For this review, use the dimensioned drawing (mm, ordinates from the lowest corner) and the shaded views. Round coordinates to 2 decimals unless told otherwise and drop trailing zeros. Order: outer loops, then holes, each group sorted by start corner. A loop starts at its lowest first (then second) coordinate and runs counter-clockwise, first axis right, second up. Notation, with made-up numbers: M 44.5,-4.75 L 78.5,-4.75 A24 ccw 78.5,18.25 Z; hole C 62,70.5 d10. An arc over 180 degrees is marked long. One line per item, written item: value. Start each with the question number.
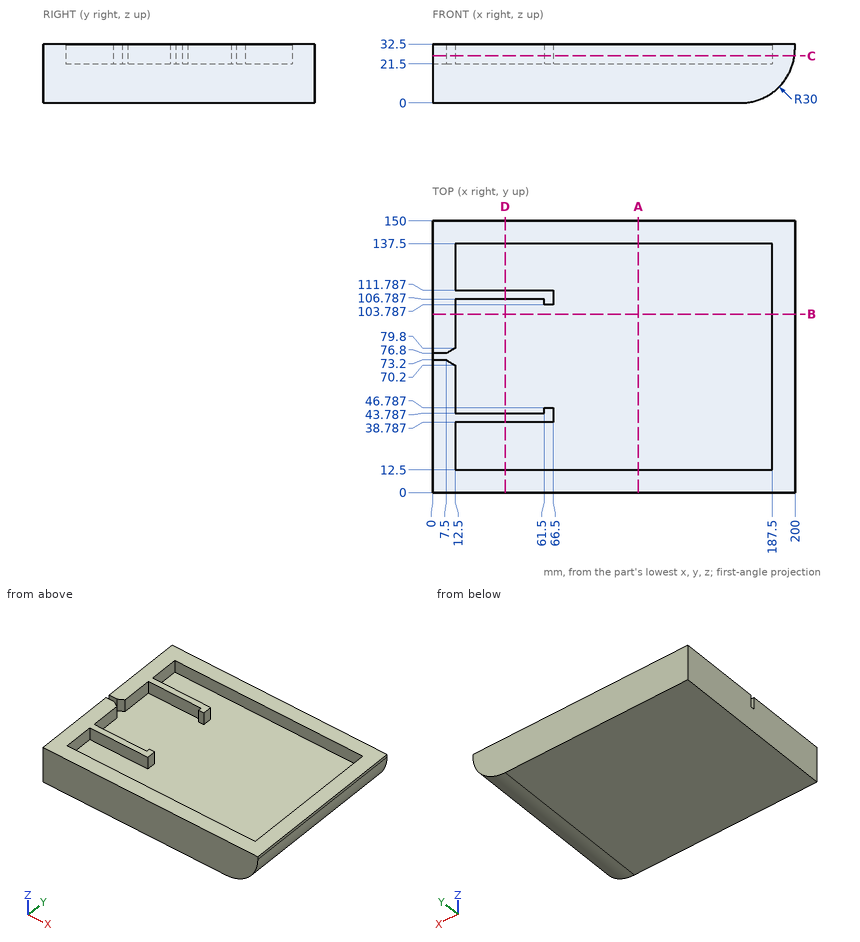
Item 1: Consider section D-D, the plane x = 40. Give the boundary of the cut face in (y, z), then the cut area to 3 significant figures.
Item 2: Clearance check with flat-ended pins moving along their axes: P1, Ø3.5, axis at y = 100, z = 24.5, coming from the +X side (1 decimal); P2, Ø3.5, axis at y = 55.5, z = 27.5, coming from the +X side; P3, Ø5.5, axis at y = 26, z = 25, coming from the +X side. State where each tip first meets the part, or that it passes through.
Item 3: Consider section A-A, the plane x = 113.5. Give the boundary of the cut face in (y, z).
Item 4: Consider section B-B, the plane y = 98.5. Give the boundary of the cut face in (x, z), then the cut area to 3 significant figures.
Item 5: Wall thickness on L1, parallel to Y at x = 50.5, z = 22.5; L2, parallel to Y at x = 64, z = 27.5; L3, parallel to X at y = 89, z = 29.5: over which ranges is each line inside the solid? List them lowest first.
Item 6: Consider section C-C, the plane z = 26. Give the boundary of the cut face in (x, y).
Computed:
1. outline: M 0,0 L 150,0 L 150,32.5 L 137.5,32.5 L 137.5,21.5 L 111.79,21.5 L 111.79,32.5 L 106.79,32.5 L 106.79,21.5 L 43.79,21.5 L 43.79,32.5 L 38.79,32.5 L 38.79,21.5 L 12.5,21.5 L 12.5,32.5 L 0,32.5 Z
1. area: 3,610 mm^2
2. P1: stops at x = 199.8
2. P2: stops at x = 199.99
2. P3: stops at x = 199.92
3. outline: M 0,0 L 150,0 L 150,32.5 L 137.5,32.5 L 137.5,21.5 L 12.5,21.5 L 12.5,32.5 L 0,32.5 Z
4. outline: M 0,0 L 170,0 A30 ccw 200,30 L 200,32.5 L 187.5,32.5 L 187.5,21.5 L 12.5,21.5 L 12.5,32.5 L 0,32.5 Z
4. area: 4,380 mm^2
5. L1: y = 0 to 12.5, 38.79 to 43.79, 106.79 to 111.79, 137.5 to 150
5. L2: y = 0 to 12.5, 38.79 to 46.79, 103.79 to 111.79, 137.5 to 150
5. L3: x = 0 to 12.5, 187.5 to 200
6. outline: M 0,0 L 199.73,0 L 199.73,150 L 0,150 L 0,76.8 L 7.5,76.8 L 12.5,79.8 L 12.5,106.79 L 61.5,106.79 L 61.5,103.79 L 66.5,103.79 L 66.5,111.79 L 12.5,111.79 L 12.5,137.5 L 187.5,137.5 L 187.5,12.5 L 12.5,12.5 L 12.5,38.79 L 66.5,38.79 L 66.5,46.79 L 61.5,46.79 L 61.5,43.79 L 12.5,43.79 L 12.5,70.2 L 7.5,73.2 L 0,73.2 Z
